The model under review builds one solid part; all positions refer to its coordinate system, in mm. A direction names the side the tool comes from. Coordinates: 2 decimals unless noted, no trailing zeros. Order: outer loops, then holes, each group sorted by start corner. A loop starts at its lowest first (then second) coordinate and runs counter-clockwise, first axis right, second up. Notation, with made-up numbers: M 9.5,85.5 L 41.5,85.5 A20 ccw 41.5,98.5 Z; hole C 45.25,72.5 d9. An arc over 180 degrees is marked long. Write each question's results on one line, items separated by ' | '.
from build123d import *

# Parameters (mm, degrees)
BOSS_EXTRU_1_DEPTH      = 15
D_GAGEMENT_M121_D       = 13.5
ENL_V_MAT_EXTRU_8_DEPTH = 33
CONG_1_R                = 5
CONG_2_R                = 5
CONG_3_R                = 5


with BuildPart() as part:
    # Esquisse1 → Boss.-Extru.1 (new body)
    with BuildSketch(Plane.XY):
        Polygon((0, 95), (207.5, 95), (207.5, 130), (332.5, 130), (332.5, 95.731450782), (539.999504611, 95.731450782), (539.999504611, 0), (0, 0), align=None)
    extrude(amount=BOSS_EXTRU_1_DEPTH)

    # Dégagement M121 (through all)
    with Locations(Plane(origin=(0, 0, 0), x_dir=(-1, 0, 0), z_dir=(0, 0, -1))):
        with Locations((-40, 47.5), (-499.999504611, 48.231450782)):
            Hole(D_GAGEMENT_M121_D / 2)

    # Esquisse20 → Enlèv. mat.-Extru.8 (cut)
    with BuildSketch(Plane(origin=(0, 0, 0), x_dir=(-1, 0, 0), z_dir=(0, 0, -1))):
        with BuildLine():
            Line((-197.499504611, 28), (-342.499504611, 28))
            ThreePointArc((-342.499504611, 28), (-362.499504611, 48), (-342.499504611, 68))
            Line((-342.499504611, 68), (-317.499504611, 68))
            Line((-317.499504611, 68), (-317.499504611, 98))
            Line((-317.499504611, 98), (-222.499504611, 98))
            Line((-222.499504611, 98), (-222.499504611, 68))
            Line((-222.499504611, 68), (-197.499504611, 68))
            ThreePointArc((-197.499504611, 68), (-177.499504611, 48), (-197.499504611, 28))
        make_face()
    extrude(amount=-ENL_V_MAT_EXTRU_8_DEPTH, mode=Mode.SUBTRACT)

    # Congé1
    cong_1_edges = [part.edges().sort_by_distance(p)[0] for p in [
        (207.5, 95, 7.5),
        (207.5, 130, 7.5),
        (332.5, 130, 7.5),
        (332.5, 95.731450782, 7.5),
    ]]
    fillet(cong_1_edges, radius=CONG_1_R)

    # Congé2
    cong_2_edges = [part.edges().sort_by_distance(p)[0] for p in [
        (317.499504611, 68, 7.5),
        (317.499504611, 98, 7.5),
        (222.499504611, 98, 7.5),
        (222.499504611, 68, 7.5),
    ]]
    fillet(cong_2_edges, radius=CONG_2_R)

    # Congé3
    cong_3_edges = [part.edges().sort_by_distance(p)[0] for p in [
        (0, 95, 7.5),
        (539.999504611, 95.731450782, 7.5),
        (539.999504611, 0, 7.5),
        (0, 0, 7.5),
    ]]
    fillet(cong_3_edges, radius=CONG_3_R)


solid = part.part
1) For faces 5 (the flat face through (222.5, 83, 7)), 6 (the flat face through (332.5, 113, 7)), 7 (the flat face through (102, 95, 7)), list the 3-axis set-ups (+Z, -Z, +X, -X, +Y, -Y) from which the entire face can be reached by the end or side of a thin tool; tool diameter is ignored.
Solutions:
face 5: +Z, -Z | face 6: +Z, -Z, +X, +Y | face 7: +Z, -Z, -X, +Y
2) Take a section at C-C on z = 11. Count the separate pieces of the cut face and the enclosed holes in it, plus the area to 3 significant figures.
Solutions:
separate pieces: 1 | enclosed holes: 3 | area: 45,600 mm2
3) For pin 1 (1 mm diameter, centred on y = 94.5, z = 5, fed in from -X); pin 2 (8 mm diameter, centred on y = 108, z = 9.5, fed in from +X); pin 3 (4.5 mm diameter, centred on y = 109.5, z = 9, fed in from -X), all flat-tipped, find the tip position at first contact; note any pin that passes through.
Solutions:
pin 1: x = 2 | pin 2: x = 332.5 | pin 3: x = 207.5
4) To check wall thickness, follow line 1 along X through (y, z) = (76.5, 12.5); line 2 along Y through (x, z) = (212, 5.25); line 3 along Y through (x, z) = (312.5, 11). State the ranges of each line that lie inside material, in increasing order.
Solutions:
line 1: 0 to 222.5, 317.5 to 540 | line 2: 0 to 28, 68 to 129.97 | line 3: 0 to 28, 98 to 130
5) Take a section at D-D on y = 118. State the section outline as (x, z) points, plus the area to 4 significant figures.
Solutions:
outline: M 207.5,0 L 332.5,0 L 332.5,15 L 207.5,15 Z | area: 1,875 mm2
6) Take a section at B-B on y = 78.5. State the section outline as (x, z) points.
Solutions:
outline: M 0,0 L 222.5,0 L 222.5,15 L 0,15 Z; M 317.5,0 L 540,0 L 540,15 L 317.5,15 Z
7) The part is to be moulded in two halves that separate along Y. For faces 1 (the flat face through (0, 47, 7)), 2 (the cylindrical face through (499.121, 54.924, 7.605)), 3 (the flat face through (269, 130, 7)), 4 (the flat face through (274, 0, 7)), say which applies: pulls with the +Y half, pulls with the -Y half, needs draft (parallel to the pull), parting line crosses it, or undercut.
Solutions:
face 1: needs draft | face 2: undercut | face 3: pulls with the +Y half | face 4: pulls with the -Y half
8) Take a section at A-A on x = 40. State the section outline as (y, z) points.
Solutions:
outline: M 0,0 L 40.75,0 L 40.75,15 L 0,15 Z; M 54.25,0 L 95,0 L 95,15 L 54.25,15 Z
